Can you work these out from the model? Positions are in its coordinate system, mm. A direction names the side the tool comes from. Give positions to 0.01 mm unless a question says otherwise; leave off trailing zeros. Order: outer loops, then holes, each group sorted by start corner. A loop starts at its lowest first (then second) coordinate and runs counter-clockwise, first axis right, second up. Notation, with made-up numbers: M 85.25,70.25 L 104.25,70.25 A12 cw 104.25,85.25 Z; hole C -27.5,-37.75 d1. An arc over 180 degrees is marked long. Answer as a JSON object with one key per item and string values.
```python
from build123d import *

# Parameters (mm, degrees)
F0_R     = 1.25
F1_DEPTH = 1


with BuildPart() as f1:
    # F0 (on Front) → F1 (new body, symmetric)
    with BuildSketch(Plane.XZ):
        with BuildLine():
            Line((1.5, -5), (1.5, 0))
            Line((1.5, 0), (1.5, 5))
            ThreePointArc((1.5, 5), (1.7592719955, 6.3462912018), (2.5, 7.5))
            Line((2.5, 7.5), (2.5, 12.5))
            Line((2.5, 12.5), (0, 12.5))
            Line((0, 12.5), (-2.5, 12.5))
            Line((-2.5, 12.5), (-2.5, 7.5))
            ThreePointArc((-2.5, 7.5), (-1.7592719955, 6.3462912018), (-1.5, 5))
            Line((-1.5, 5), (-1.5, 0))
            Line((-1.5, 0), (-1.5, -5))
            ThreePointArc((-1.5, -5), (-1.7592719955, -6.3462912018), (-2.5, -7.5))
            Line((-2.5, -7.5), (-2.5, -12.5))
            Line((-2.5, -12.5), (0, -12.5))
            Line((0, -12.5), (2.5, -12.5))
            Line((2.5, -12.5), (2.5, -7.5))
            ThreePointArc((2.5, -7.5), (1.7592719955, -6.3462912018), (1.5, -5))
        make_face()
        with Locations((0, -10)):
            Circle(F0_R, mode=Mode.SUBTRACT)
        with Locations((0, 10)):
            Circle(F0_R, mode=Mode.SUBTRACT)
    extrude(amount=F1_DEPTH, both=True)


solid = f1.part
```
1) For faces 5 (the face through (-1.766, -0.014, 6.364)), 6 (the face through (1.5, 0, 0)), 7 (the face through (0.672, 0.014, -8.946)), which set-ups out of +Z, -Z, +X, -X, +Y, -Y let a thin tool reach every point of the face, with its end or its side?
Results found:
{"face 5": "-X, +Y, -Y", "face 6": "+X, +Y, -Y", "face 7": "+Y, -Y"}
2) I'm going to push flat-ended pins straight in: pin 1 Ø1.5 at (x, z) = (0, 10) entering from -Y; pin 2 Ø1 at (y, z) = (-0.5, 5) entering from +X. Where does each tip first touch, or does it pass through?
Results found:
{"pin 1": "passes through", "pin 2": "stops at x = 1.53"}
3) I need wall thicknesses on L1, parallel to Z at x = 0, y = -0.45; L2, parallel to X at y = 0.75, z = 3.5; L3, parallel to Z at x = -1.95, y = -0.8. Which ranges of each line are inside material? Lowest first, please.
Results found:
{"L1": "z = -12.5 to -11.25, -8.75 to 8.75, 11.25 to 12.5", "L2": "x = -1.5 to 1.5", "L3": "z = -12.5 to -6.75, 6.75 to 12.5"}
4) I want a section at B-B on z = -10. Write out the boundary of the cut face in (x, y).
Results found:
{"outline": "M -2.5,-1 L -1.25,-1 L -1.25,1 L -2.5,1 Z; M 1.25,-1 L 2.5,-1 L 2.5,1 L 1.25,1 Z"}
5) I want a section at A-A on x = 0. Write out the boundary of the cut face in (y, z), and give its area (3 significant figures).
Results found:
{"outline": "M -1,-12.5 L 1,-12.5 L 1,-11.25 L -1,-11.25 Z; M -1,-8.75 L 1,-8.75 L 1,8.75 L -1,8.75 Z; M -1,11.25 L 1,11.25 L 1,12.5 L -1,12.5 Z", "area": "40.0 mm²"}
6) Thinking about a two-plate mould opening in X: for faces 1 (the face through (1.752, -0.014, 6.328)), 2 (the face through (-1.752, -0.014, -6.328)), 3 (the face through (-0.16, 0.01, 11.24)), 4 (the face through (0, 0, 12.5)), which applies, pulls with the +X half, pulls with the -X half, needs draft (parallel to the pull), parting line crosses it, or undercut?
Results found:
{"face 1": "pulls with the +X half", "face 2": "pulls with the -X half", "face 3": "undercut", "face 4": "needs draft"}
7) I want a section at C-C on y = -0.45. Write out the boundary of the cut face in (x, z) (3 decimals).
Results found:
{"outline": "M -2.5,-12.5 L 2.5,-12.5 L 2.5,-7.5 A3.625 cw 1.5,-5 L 1.5,5 A3.625 cw 2.5,7.5 L 2.5,12.5 L -2.5,12.5 L -2.5,7.5 A3.625 cw -1.5,5 L -1.5,-5 A3.625 cw -2.5,-7.5 Z; hole C 0,-10 d2.5; hole C 0,10 d2.5"}
8) I want a section at D-D on z = -1.25. Write out the boundary of the cut face in (x, y), and give its area (3 significant figures).
Results found:
{"outline": "M -1.5,-1 L 1.5,-1 L 1.5,1 L -1.5,1 Z", "area": "6.00 mm²"}
